Can you work these out from the drawing? Everything is in mm from the part's minimum corner. A direction names the side the tool comes from. Round coordinates to 2 decimals unless told otherwise and drop trailing zeros. Order: outer loops, then holes, each group sorted by start corner. A loop starts at its lowest first (then second) coordinate and runs counter-clockwise, first axis right, second up. Notation, with made-up numbers: (1, 83) -> (47, 83) arc R12 cw to (47, 95) -> close; hole circle Ø9 at (25, -22). An arc over 180 degrees is marked (long way). One line per item, written item: value.
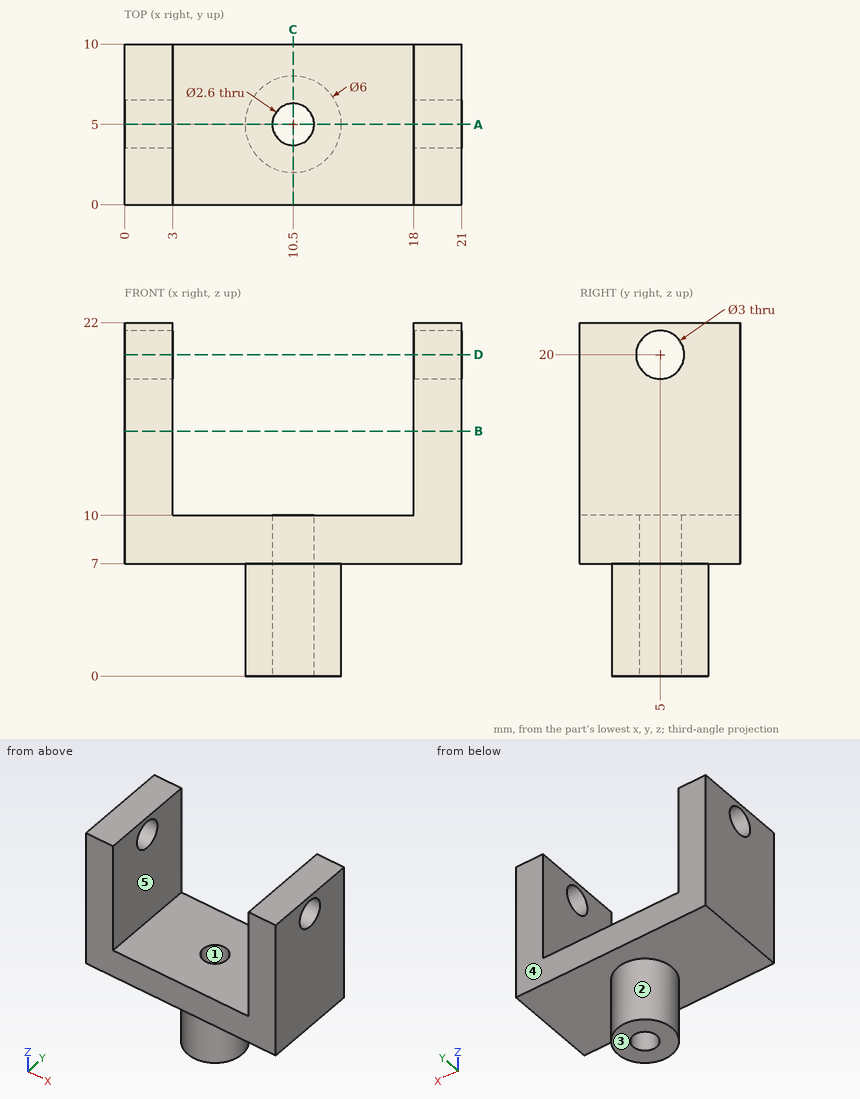
Q1. I want a section at A-A on y = 5. Write out the boundary of the cut face in (x, z), then the cut area to 3 significant figures.
Answers:
outline: (0, 7) -> (7.5, 7) -> (7.5, 0) -> (9.2, 0) -> (9.2, 10) -> (3, 10) -> (3, 18.5) -> (0, 18.5) -> close; (0, 21.5) -> (3, 21.5) -> (3, 22) -> (0, 22) -> close; (11.8, 0) -> (13.5, 0) -> (13.5, 7) -> (21, 7) -> (21, 18.5) -> (18, 18.5) -> (18, 10) -> (11.8, 10) -> close; (18, 21.5) -> (21, 21.5) -> (21, 22) -> (18, 22) -> close
area: 133 mm2
Q2. I want a section at D-D on z = 20. Write out the boundary of the cut face in (x, y), then the cut area to 3 significant figures.
Answers:
outline: (0, 0) -> (3, 0) -> (3, 3.5) -> (0, 3.5) -> close; (0, 6.5) -> (3, 6.5) -> (3, 10) -> (0, 10) -> close; (18, 0) -> (21, 0) -> (21, 3.5) -> (18, 3.5) -> close; (18, 6.5) -> (21, 6.5) -> (21, 10) -> (18, 10) -> close
area: 42.0 mm2
Q3. I want a section at B-B on z = 15.25. Write out the boundary of the cut face in (x, y), then the cut area to 3 significant figures.
Answers:
outline: (0, 0) -> (3, 0) -> (3, 10) -> (0, 10) -> close; (18, 0) -> (21, 0) -> (21, 10) -> (18, 10) -> close
area: 60.0 mm2
Q4. I need wall thicknesses on line 1 along X through (y, z) = (7.25, 13.5); line 2 along Y through (x, z) = (18.7, 20); line 3 along Y through (x, z) = (10.5, 6). Which ranges of each line are inside material? Lowest first, please.
Answers:
line 1: 0 to 3, 18 to 21
line 2: 0 to 3.5, 6.5 to 10
line 3: 2 to 3.7, 6.3 to 8
Q5. I want a section at C-C on x = 10.5. Write out the boundary of the cut face in (y, z), then the cut area to 3 significant figures.
Answers:
outline: (0, 7) -> (2, 7) -> (2, 0) -> (3.7, 0) -> (3.7, 10) -> (0, 10) -> close; (6.3, 0) -> (8, 0) -> (8, 7) -> (10, 7) -> (10, 10) -> (6.3, 10) -> close
area: 46.0 mm2
Q6. If we mould it in two halves opening along X, with no side actions, what happens to the marked faces 1, 2 and 3? For each: pulls with the +X half, pulls with the -X half, needs draft (parallel to the pull), parting line crosses it, or undercut.
Answers:
face 1: undercut
face 2: parting line crosses it
face 3: needs draft
Q7. Which directions (+Z, -Z, +X, -X, +Y, -Y) give clear straight access to the entire face, cutting with the end or side of a thin tool? Please do the marked faces 4 and 5.
Answers:
face 4: +Z, -Z, +X, -X, +Y
face 5: +Z, +Y, -Y
Q8. For P1, Ø3, axis at x = 10, y = 7.5, coming from the +Z side, with a flat end and sliding along its axis, tell me the tip position at first contact or that it passes through.
Answers:
P1: z = 10
